Verification items for the finished model (mm, model axes). A direction names the side the tool comes from. Round coordinates to 2 decimals unless told otherwise and drop trailing zeros. Write each loop counter-clockwise with the first axis right and the second up, starting at its lowest first coordinate (ties: lowest second). Pieces come first, ordered by that corner, then holes. Notation, with made-up numbers: (16.5, -35.75) -> (75.5, -35.75) arc R20 ccw to (75.5, -0.75) -> close; hole circle Ø9 at (-18, -15). An arc over 180 degrees is marked (long way). Answer as a JSON object with one key per item and string values. Group by question number.
(1) Sectioned sample at D-D on y = -3. Record the cut outline in (x, z).
(2) Sectioned sample at B-B on z = 6.25. Record the cut outline in (x, y).
(3) Draft check along X on faces 4 (the face through (-45, 11, 10)), 5 (the face through (-44.69, 18, 5)), 6 (the face through (-50.799, 17, 5)). Enter one of: released by +X, released by -X, zero draft, split by the parting line, or undercut.
(4) Scan lines: L1, parallel to Y at x = -44, z = 8.25; L2, parallel to X at y = 34.5, z = 2; L3, parallel to Y at x = -21.5, z = 4. Record each from-to range of solid material in increasing order. Write a range as from..to.
(5) Gauge pin test, flat ends, axial feed: pin 1 Ø3 at (y, z) = (18, 5) entering from +X; pin 2 Ø12 at (x, y) = (-41, 35) entering from -Z. Record the tip position at first contact, or that the pin passes through.
(6) Sectioned sample at A-A on x = -28. Record the cut outline in (y, z), and give its area (3 significant figures).
(7) Sectioned sample at C-C on y = 19. Record the cut outline in (x, z).
(8) Set-up check for faces 1 (the face through (-48, 19.807, 5)), 2 (the face through (-51.761, 18, 5)), 3 (the face through (-30, -15.285, 5)): record each of +Z, -Z, +X, -X, +Y, -Y from which the full face is reachable in a straight line by a thin tool's end or side.
```python
from build123d import *

# Parameters (mm, degrees)
BOSS_EXTRUDE1_DEPTH     = 10
SKETCH2_W               = 5
SKETCH2_H               = 5.5
CUT_EXTRUDE2_DEPTH      = 11
CUT_EXTRUDE2_DEPTH_BACK = 10


with BuildPart() as part:
    # Sketch1 → Boss-Extrude1 (new body)
    with BuildSketch(Plane.XY):
        Polygon((-15.00519424, 49.714572154), (-44.689605678, 49.714572154), (-44.689605678, -15.285427846), (-14.689605678, -15.285427846), (-21.76067349, -22.356495658), (-51.76067349, -22.356495658), (-51.76067349, -18.214360034), (-51.76067349, 56.470051403), (-21.76067349, 56.470051403), align=None)
    extrude(amount=BOSS_EXTRUDE1_DEPTH)

    # Sketch2 → Cut-Extrude2 (cut, two sides)
    with BuildSketch(Plane.XY) as cut_extrude2_sk:
        with Locations((-48.298710813, 17.056777872)):
            Rectangle(SKETCH2_W, SKETCH2_H)
    extrude(amount=CUT_EXTRUDE2_DEPTH, mode=Mode.SUBTRACT)
    extrude(cut_extrude2_sk.sketch, amount=-CUT_EXTRUDE2_DEPTH_BACK, mode=Mode.SUBTRACT)


solid = part.part
```
Computed values:
{
 "1": {"outline": "(-51.76, 0) -> (-44.69, 0) -> (-44.69, 10) -> (-51.76, 10) -> close"},
 "2": {"outline": "(-51.76, -22.36) -> (-21.76, -22.36) -> (-14.69, -15.29) -> (-44.69, -15.29) -> (-44.69, 49.71) -> (-15.01, 49.71) -> (-21.76, 56.47) -> (-51.76, 56.47) -> close; hole (-50.8, 14.31) -> (-45.8, 14.31) -> (-45.8, 19.81) -> (-50.8, 19.81) -> close"},
 "3": {"face 4": "zero draft", "face 5": "released by +X", "face 6": "undercut"},
 "4": {"L1": "-22.36..-15.29, 49.71..56.47", "L2": "-51.76..-44.69", "L3": "-22.1..-15.29, 49.71..56.21"},
 "5": {"pin 1": "x = -44.69", "pin 2": "z = 0"},
 "6": {"outline": "(-22.36, 0) -> (-15.29, 0) -> (-15.29, 10) -> (-22.36, 10) -> close; (49.71, 0) -> (56.47, 0) -> (56.47, 10) -> (49.71, 10) -> close", "area": "138 mm2"},
 "7": {"outline": "(-51.76, 0) -> (-50.8, 0) -> (-50.8, 10) -> (-51.76, 10) -> close; (-45.8, 0) -> (-44.69, 0) -> (-44.69, 10) -> (-45.8, 10) -> close"},
 "8": {"face 1": "+Z, -Z", "face 2": "+Z, -Z, -X, +Y, -Y", "face 3": "+Z, -Z, +X"}
}
